Geometry check sheet. Reference: the model listing, model coordinates, mm. A direction names the side the tool comes from. Round coordinates to 2 decimals unless told otherwise and drop trailing zeros. Order: outer loops, then holes, each group sorted by start corner. A loop starts at its lowest first (then second) coordinate and runs counter-clockwise, first axis right, second up. Notation, with made-up numbers: (35.5, -29) - (93.5, -29) arc R5 ccw to (93.5, -23) - close; hole circle Ø2 at (65.25, 19.25). An arc over 180 degrees is marked (long way). Use a Markdown table: item, result. Add a question column.
(1) Section check A-A on z = -13. Record the boundary of the cut face in (x, y).
(2) Thickness scan on line 1 along Z through (x, y) = (7.5, 2.3); line 2 along X through (y, z) = (1.6, -13); line 3 along X through (y, z) = (2.1, -29.5). Record the ranges inside material, lowest first. Write a range as [from, to].
(3) Section check C-C on y = 0.8. Record the boundary of the cut face in (x, z).
(4) Gauge pin test, flat end, axial feed: P1, Ø2, axis at x = 7.5, z = -57.5, coming from the +Y side. Record the tip position at first contact, or that the pin passes through.
(5) Mould release check, pull along Z, two halves, no side actions. Record for faces 1 (the face through (12.5, 2, -35)), 2 (the face through (7, 1, 0)), 3 (the face through (7, 1, -110)), 4 (the face through (7, 0, -56)): released by +Z, released by -Z, zero draft, split by the parting line, or undercut.
(6) Access from +Z, -Z, +X, -X, +Y, -Y to the whole of each face (thin tool, end or side, straight path). Record for faces 5 (the face through (15, 1, -54)), 6 (the face through (7.6, 1.5, -23)).
(7) Section check B-B on x = 4.5. Record the boundary of the cut face in (y, z), then the cut area to 4 significant figures.
```python
from build123d import *

# Parameters (mm, degrees)
SKETCH_1_W          = 15
SKETCH_1_H          = 110
EXTRUDE_1_DEPTH     = 3
FILLET_1_R          = 1
SKETCH_2_R          = 1.25
CUT_EXTRUDE_1_DEPTH = 3
CUT_EXTRUDE_2_DEPTH = 10


with BuildPart() as part:
    # 草图1 → 凸台-拉伸1 (new body)
    with BuildSketch(Plane(origin=(0, 0, 0), x_dir=(1, 0, 0), z_dir=(0, 1, 0))):
        with Locations((7.5, 55)):
            Rectangle(SKETCH_1_W, SKETCH_1_H)
    extrude(amount=EXTRUDE_1_DEPTH)

    # 圆角1
    fillet_1_edges = [part.edges().sort_by_distance(p)[0] for p in [
        (0, 1.5, -110),
        (15, 1.5, -110),
        (15, 1.5, 0),
        (0, 1.5, 0),
    ]]
    fillet(fillet_1_edges, radius=FILLET_1_R)

    # 草图2 → 切除-拉伸1 (cut)
    with BuildSketch(Plane(origin=(0, 3, 0), x_dir=(1, 0, 0), z_dir=(0, 1, 0))):
        with Locations((7.5, 13)):
            Circle(SKETCH_2_R)
        with Locations((7.5, 57.5)):
            Circle(SKETCH_2_R)
    extrude(amount=-CUT_EXTRUDE_1_DEPTH, mode=Mode.SUBTRACT)

    # 草图3 → 切除-拉伸2 (cut)
    with BuildSketch(Plane(origin=(0, 3, 0), x_dir=(1, 0, 0), z_dir=(0, 1, 0))):
        with BuildLine():
            Line((12.5, 42.5), (12.5, 28))
            ThreePointArc((12.5, 28), (7.5, 23), (2.5, 28))
            Line((2.5, 28), (2.5, 42.5))
            ThreePointArc((2.5, 42.5), (7.5, 47.5), (12.5, 42.5))
        make_face()
    extrude(amount=-CUT_EXTRUDE_2_DEPTH, mode=Mode.SUBTRACT)


solid = part.part
```
Check sheet entries:
| question | item | result |
|---|---|---|
| 1 | outline | (0, 0) - (6.25, 0) - (6.25, 3) - (0, 3) - close; (8.75, 0) - (15, 0) - (15, 3) - (8.75, 3) - close |
| 2 | line 1 | z = [-110, -58.75], [-56.25, -47.5], [-23, -14.25], [-11.75, 0] |
| 2 | line 2 | x = [0, 6.25], [8.75, 15] |
| 2 | line 3 | x = [0, 2.5], [12.5, 15] |
| 3 | outline | (0, -109) arc R1 ccw to (1, -110) - (14, -110) arc R1 ccw to (15, -109) - (15, -1) arc R1 ccw to (14, 0) - (1, 0) arc R1 ccw to (0, -1) - close; hole (2.5, -42.5) arc R5 ccw to (12.5, -42.5) - (12.5, -28) arc R5 ccw to (2.5, -28) - close; hole circle Ø2.5 at (7.5, -57.5); hole circle Ø2.5 at (7.5, -13) |
| 4 | P1 | passes through |
| 5 | face 1 | undercut |
| 5 | face 2 | released by +Z |
| 5 | face 3 | released by -Z |
| 5 | face 4 | zero draft |
| 6 | face 5 | +Z, -Z, +X, +Y, -Y |
| 6 | face 6 | +Y, -Y |
| 7 | outline | (0, -110) - (3, -110) - (3, -46.5) - (0, -46.5) - close; (0, -24) - (3, -24) - (3, 0) - (0, 0) - close |
| 7 | area | 262.5 mm2 |
